from build123d import *

# Parameters (mm, degrees)
F1_DEPTH    = 15
F2_T1_DEPTH = 15.9585845768


# Not quite as in the source:
# - a fillet or chamfer that OpenCascade refuses, or shapes differently, is made with other operations: its cross-section is extruded or revolved along the edge and cut away or added


with BuildPart() as f1:
    # F0 (on Top) → F1 (new body)
    with BuildSketch(Plane.XY):
        with BuildLine():
            ThreePointArc((2.9247837365, -0.6675628019), (3.7405193144, 0.3530547619), (4.9127228226, 0.9301368008))
            ThreePointArc((4.9127228226, 0.9301368008), (4.8746395609, 1.1126046698), (4.8297815528, 1.2935262471))
            ThreePointArc((4.8297815528, 1.2935262471), (3.5232761722, 1.3048591573), (2.3454944474, 1.8704694056))
            ThreePointArc((2.3454944474, 1.8704694056), (2.0561463183, 3.1445818043), (2.3358223454, 4.420852177))
            ThreePointArc((2.3358223454, 4.420852177), (2.1694186956, 4.5048443395), (2, 4.582575695))
            ThreePointArc((2, 4.582575695), (1.1765467932, 3.5681746103), (0, 3))
            ThreePointArc((0, 3), (-1.1765467932, 3.5681746103), (-2, 4.582575695))
            ThreePointArc((-2, 4.582575695), (-2.1694186956, 4.5048443395), (-2.3358223454, 4.420852177))
            ThreePointArc((-2.3358223454, 4.420852177), (-2.0561463183, 3.1445818043), (-2.3454944474, 1.8704694056))
            ThreePointArc((-2.3454944474, 1.8704694056), (-3.5232761722, 1.3048591573), (-4.8297815528, 1.2935262471))
            ThreePointArc((-4.8297815528, 1.2935262471), (-4.8746395609, 1.1126046698), (-4.9127228226, 0.9301368008))
            ThreePointArc((-4.9127228226, 0.9301368008), (-3.7405193144, 0.3530547619), (-2.9247837365, -0.6675628019))
            ThreePointArc((-2.9247837365, -0.6675628019), (-3.2169067319, -1.9410418555), (-4.0226390868, -2.9695748479))
            ThreePointArc((-4.0226390868, -2.9695748479), (-3.9091574123, -3.1174490093), (-3.7902428131, -3.2609905577))
            ThreePointArc((-3.7902428131, -3.2609905577), (-2.608204974, -2.7043297172), (-1.3016512174, -2.7029066037))
            ThreePointArc((-1.3016512174, -2.7029066037), (-0.4881409094, -3.725298761), (-0.1863673415, -4.9965255142))
            ThreePointArc((-0.1863673415, -4.9965255142), (0, -5), (0.1863673415, -4.9965255142))
            ThreePointArc((0.1863673415, -4.9965255142), (0.4881409094, -3.725298761), (1.3016512174, -2.7029066037))
            ThreePointArc((1.3016512174, -2.7029066037), (2.608204974, -2.7043297172), (3.7902428131, -3.2609905577))
            ThreePointArc((3.7902428131, -3.2609905577), (3.9091574123, -3.1174490093), (4.0226390868, -2.9695748479))
            ThreePointArc((4.0226390868, -2.9695748479), (3.2169067319, -1.9410418555), (2.9247837365, -0.6675628019))
        make_face()
    extrude(amount=F1_DEPTH)

    # F2: fillet of radius 0.2 on 14 edges, made by hand

    # F2_s2 → F2_t1 (cut)
    with BuildSketch(Plane.XY.offset(-0.4792922884)):
        with BuildLine():
            ThreePointArc((-3.9124710062, -3.1132893578), (-3.785825601, -3.1865171636), (-3.6432075854, -3.1539369268))
            ThreePointArc((-3.6432075854, -3.1539369268), (-3.7175366677, -3.2063492126), (-3.7902428131, -3.2609905577))
            ThreePointArc((-3.7902428131, -3.2609905577), (-3.8520648952, -3.1877258419), (-3.9124710062, -3.1132893578))
        make_face()
        with BuildLine():
            ThreePointArc((-3.8855510977, -2.8500477743), (-3.949049974, -2.9818402738), (-3.905839396, -3.121605134))
            ThreePointArc((-3.905839396, -3.121605134), (-3.9649679778, -3.0461498543), (-4.0226390868, -2.9695748479))
            ThreePointArc((-4.0226390868, -2.9695748479), (-3.9531890749, -2.9108504406), (-3.8855510977, -2.8500477743))
        make_face()
        with BuildLine():
            ThreePointArc((-0.1943444075, -4.814821897), (-0.1308957841, -4.946638597), (0.0053181385, -4.9999971717))
            ThreePointArc((0.0053181385, -4.9999971717), (-0.0905412424, -4.9991801611), (-0.1863673415, -4.9965255142))
            ThreePointArc((-0.1863673415, -4.9965255142), (-0.1889785578, -4.9056132393), (-0.1943444075, -4.814821897))
        make_face()
        with BuildLine():
            ThreePointArc((-0.0053181385, -4.9999971717), (0.1308957841, -4.946638597), (0.1943444075, -4.814821897))
            ThreePointArc((0.1943444075, -4.814821897), (0.1889785578, -4.9056132393), (0.1863673415, -4.9965255142))
            ThreePointArc((0.1863673415, -4.9965255142), (0.0905412424, -4.9991801611), (-0.0053181385, -4.9999971717))
        make_face()
        with BuildLine():
            ThreePointArc((3.6432075854, -3.1539369268), (3.785825601, -3.1865171636), (3.9124710062, -3.1132893578))
            ThreePointArc((3.9124710062, -3.1132893578), (3.8520648952, -3.1877258419), (3.7902428131, -3.2609905577))
            ThreePointArc((3.7902428131, -3.2609905577), (3.7175366677, -3.2063492126), (3.6432075854, -3.1539369268))
        make_face()
        with BuildLine():
            ThreePointArc((3.8855510977, -2.8500477743), (3.949049974, -2.9818402738), (3.905839396, -3.121605134))
            ThreePointArc((3.905839396, -3.121605134), (3.9649679778, -3.0461498543), (4.0226390868, -2.9695748479))
            ThreePointArc((4.0226390868, -2.9695748479), (3.9531890749, -2.9108504406), (3.8855510977, -2.8500477743))
        make_face()
        with BuildLine():
            ThreePointArc((4.7373499587, 0.8819268779), (4.8517430918, 0.973116687), (4.8734534064, 1.1177888421))
            ThreePointArc((4.8734534064, 1.1177888421), (4.8939875989, 1.024151054), (4.9127228226, 0.9301368008))
            ThreePointArc((4.9127228226, 0.9301368008), (4.8246709586, 0.9073611688), (4.7373499587, 0.8819268779))
        make_face()
        with BuildLine():
            ThreePointArc((4.8758202007, 1.1074192388), (4.7934889875, 1.228344594), (4.6508585605, 1.2608704528))
            ThreePointArc((4.6508585605, 1.2608704528), (4.7405675882, 1.2758421104), (4.8297815528, 1.2935262471))
            ThreePointArc((4.8297815528, 1.2935262471), (4.8536929553, 1.2006934229), (4.8758202007, 1.1074192388))
        make_face()
        with BuildLine():
            ThreePointArc((2.2641711887, 4.2536817555), (2.2641990769, 4.3999738244), (2.1646259913, 4.5071492451))
            ThreePointArc((2.1646259913, 4.5071492451), (2.2506378215, 4.4648213174), (2.3358223454, 4.420852177))
            ThreePointArc((2.3358223454, 4.420852177), (2.2987296122, 4.3378100833), (2.2641711887, 4.2536817555))
        make_face()
        with BuildLine():
            ThreePointArc((2.1742089456, 4.5025343375), (2.0283330241, 4.5135609289), (1.913974667, 4.4223275119))
            ThreePointArc((1.913974667, 4.4223275119), (1.9582020177, 4.5017995299), (2, 4.582575695))
            ThreePointArc((2, 4.582575695), (2.0874881401, 4.543390063), (2.1742089456, 4.5025343375))
        make_face()
        with BuildLine():
            ThreePointArc((-1.913974667, 4.4223275119), (-2.0283330241, 4.5135609289), (-2.1742089456, 4.5025343375))
            ThreePointArc((-2.1742089456, 4.5025343375), (-2.0874881401, 4.543390063), (-2, 4.582575695))
            ThreePointArc((-2, 4.582575695), (-1.9582020177, 4.5017995299), (-1.913974667, 4.4223275119))
        make_face()
        with BuildLine():
            ThreePointArc((-2.1646259913, 4.5071492451), (-2.2641990769, 4.3999738244), (-2.2641711887, 4.2536817555))
            ThreePointArc((-2.2641711887, 4.2536817555), (-2.2987296122, 4.3378100833), (-2.3358223454, 4.420852177))
            ThreePointArc((-2.3358223454, 4.420852177), (-2.2506378215, 4.4648213174), (-2.1646259913, 4.5071492451))
        make_face()
        with BuildLine():
            ThreePointArc((-4.8734534064, 1.1177888421), (-4.8517430918, 0.973116687), (-4.7373499587, 0.8819268779))
            ThreePointArc((-4.7373499587, 0.8819268779), (-4.8246709586, 0.9073611688), (-4.9127228226, 0.9301368008))
            ThreePointArc((-4.9127228226, 0.9301368008), (-4.8939875989, 1.024151054), (-4.8734534064, 1.1177888421))
        make_face()
        with BuildLine():
            ThreePointArc((-4.6508585605, 1.2608704528), (-4.7934889875, 1.228344594), (-4.8758202007, 1.1074192388))
            ThreePointArc((-4.8758202007, 1.1074192388), (-4.8536929553, 1.2006934229), (-4.8297815528, 1.2935262471))
            ThreePointArc((-4.8297815528, 1.2935262471), (-4.7405675882, 1.2758421104), (-4.6508585605, 1.2608704528))
        make_face()
    extrude(amount=F2_T1_DEPTH, mode=Mode.SUBTRACT)


solid = f1.part
Geometry check sheet. Reference: the model listing, model coordinates, mm. A direction names the side the tool comes from. Give positions to 0.01 mm unless a question says otherwise; leave off trailing zeros. Write each loop counter-clockwise with the first axis right and the second up, starting at its lowest first coordinate (ties: lowest second). Pieces come first, ordered by that corner, then holes. Notation, with made-up numbers: (4, -16.75) - (44, -16.75) arc R15 cw to (44, -1.75) - close; hole circle Ø2 at (15, 16.25). An arc over 180 degrees is marked (long way). Put each result on its own line as item: value.
1. Thickness scan on line 1 (X direction, y = -3, z = 5.75); line 2 (Y direction, x = -3.5, z = 1.75); line 3 (Y direction, x = -2, z = 3). Record the ranges inside material, lowest first.
Ans:
line 1: x = -3.95 to -3.39, -0.98 to 0.98, 3.39 to 3.95
line 2: y = -3.06 to -2.42, 0.14 to 1.31
line 3: y = -2.63 to 4.5
2. Sectioned sample at B-B, the plane x = 1.5. Enter the section's corners in (y, z), plus the area to 3 significant figures.
Ans:
outline: (-2.67, 0) - (3.87, 0) - (3.87, 15) - (-2.67, 15) - close
area: 98.0 mm²
3. Go/stop test with flat-tipped pins: pin 1 (3 mm diameter, centred on y = 3.5, z = 11.5, fed in from +X); pin 2 (1.5 mm diameter, centred on y = 0, z = 10, fed in from -X). Record where each tip stops, or that it passes through.
Ans:
pin 1: stops at x = 2.29
pin 2: stops at x = -4.39
4. Set-up check for faces 1 (the cylindrical face through (3.186, -1.874, 7.395)), 2 (the cylindrical face through (-1.09, 3.5, 7.4)), 3 (the cylindrical face through (-3.684, 0.306, 7.395)): record each of +Z, -Z, +X, -X, +Y, -Y from which the full face is reachable in a straight line by a thin tool's end or side.
Ans:
face 1: +Z, -Z, +X
face 2: +Z, -Z, +Y
face 3: +Z, -Z, -X
5. Sectioned sample at A-A, the plane z = 14.25. Enter the section's corners in (x, y), plus the area to 3 significant figures.
Ans:
outline: (-4.87, 1.11) arc R0.2 ccw to (-4.74, 0.88) arc R3 cw to (-2.92, -0.67) arc R3 cw to (-3.89, -2.85) arc R0.2 ccw to (-3.91, -3.12) arc R0.2 ccw to (-3.64, -3.15) arc R3 cw to (-1.3, -2.7) arc R3 cw to (-0.19, -4.81) arc R0.2 ccw to (0, -5) arc R0.2 ccw to (0.19, -4.81) arc R3 cw to (1.3, -2.7) arc R3 cw to (3.64, -3.15) arc R0.2 ccw to (3.91, -3.12) arc R0.2 ccw to (3.89, -2.85) arc R3 cw to (2.92, -0.67) arc R3 cw to (4.74, 0.88) arc R0.2 ccw to (4.87, 1.11) arc R0.2 ccw to (4.65, 1.26) arc R3 cw to (2.35, 1.87) arc R3 cw to (2.26, 4.25) arc R0.2 ccw to (2.17, 4.5) arc R0.2 ccw to (1.91, 4.42) arc R3 cw to (0, 3) arc R3 cw to (-1.91, 4.42) arc R0.2 ccw to (-2.17, 4.5) arc R0.2 ccw to (-2.26, 4.25) arc R3 cw to (-2.35, 1.87) arc R3 cw to (-4.65, 1.26) arc R0.2 ccw to start
area: 41.6 mm²
6. Sectioned sample at C-C, the plane y = -4. Enter the section's corners in (x, z).
Ans:
outline: (-0.37, 0) - (0.37, 0) - (0.37, 15) - (-0.37, 15) - close
7. Draft check along Y on faces 4 (the cylindrical face through (0.5, -3.7, 7.4)), 5 (the cylindrical face through (3.452, 1.322, 7.395)), 6 (the cylindrical face through (-3.17, -1.84, 7.4)), 7 (the cylindrical face through (-2.057, 3.071, 7.395)). Enter one of: +Y half, -Y half, draft (parallel to the pull), parting line (faces both ways), or undercut.
Ans:
face 4: -Y half
face 5: +Y half
face 6: undercut
face 7: undercut
